from build123d import *


with BuildPart() as f5:
    # F2 (on offset) → F5 section 0
    with BuildSketch(Plane.XY.offset(2), mode=Mode.PRIVATE) as f5_s0:
        Polygon((9.893138, -2.562072), (8.171379, 6.137341), (0.296405, 10.215211), (-7.801768, 6.600819), (-10.025051, -1.984125), (-4.699266, -9.074982), (4.165162, -9.332193), align=None)
    loft([Vertex(0.172753, -0.103171, 12), f5_s0.sketch])

    # F0 (on Top) → F6 section 0
    with BuildSketch(Plane.XY):
        Polygon((7.732626, -1.753436), (6.192105, 4.952361), (-0.011197, 7.928929), (-6.206068, 4.934852), (-7.727643, -1.775269), (-3.430145, -7.148577), (3.450322, -7.13886), align=None)
    # F5_face (on face) → F6 section 1
    with BuildSketch(Plane(origin=(0, 0, 2), x_dir=(1, 0, 0), z_dir=(0, 0, -1))):
        Polygon((9.893138, 2.562072), (4.165162, 9.332193), (-4.699266, 9.074982), (-10.025051, 1.984125), (-7.801768, -6.600819), (0.296405, -10.215211), (8.171379, -6.137341), align=None)
    loft()


solid = f5.part
Geometry: final body of the model. Coordinates: model frame, mm. Round coordinates to 2 decimals unless told otherwise and drop trailing zeros. Loops run counter-clockwise (first coordinate to the right, second up) from the corner with the lowest first, then second, coordinate; pieces in that order, holes last. Notation, with made-up numbers: (-24.75, 1) - (10.25, 1) arc R19 ccw to (10.25, 7) - close; hole circle Ø2 at (-38, 26.5). An arc over 180 degrees is marked (long way). Write each question's results on one line, items separated by ' | '. Start each with the question number.
1) First-contact query: P1, Ø2, axis at x = -3, z = 8.5, coming from the -Y side; P2, Ø2, axis at x = -0.5, y = -1, coming from the +Z side; P3, Ø4, axis at x = 2.5, y = 7, coming from the +Z side. Flat tips, straight axial feed; report the tip coordinate or a pass-through.
2) Cut plane B-B on z = 10.25. Return loops of the section in (x, y), then the cut area to 3 significant figures.
3) Line query: probe 1 along Z at (x, y) = (-5.25, 0.75); probe 2 along X at (y, z) = (-5.25, 1.5); probe 3 along Z at (x, y) = (-3.75, -5). Output: solid intervals per line, ascending. Write a range as [from, to].
4) Cut plane A-A on z = 7. Return loops of the section in (x, y).
5) Mould query, pull axis X, two halves, no side actions, for faces 1 (the face through (0, 0, 0)), 2 (the face through (2.67, 5.02, 5.82)), 3 (the face through (-2.2, 5.2, 5.8)). Classes: released by +X, released by -X, zero draft, split by the parting line, or undercut.
Verdict:
1) P1: stops at y = -3.33 | P2: stops at z = 11.88 | P3: stops at z = 6.17
2) outline: (-1.61, -0.43) - (-0.68, -1.67) - (0.87, -1.72) - (1.87, -0.53) - (1.57, 0.99) - (0.19, 1.7) - (-1.22, 1.07) - close | area: 8.75 mm2
3) probe 1: z = [0, 6.19] | probe 2: x = [-6.93, 6.94] | probe 3: z = [0, 5.45]
4) outline: (-4.93, -1.04) - (-2.26, -4.59) - (2.17, -4.72) - (5.03, -1.33) - (4.17, 3.02) - (0.23, 5.06) - (-3.81, 3.25) - close
5) face 1: zero draft | face 2: released by +X | face 3: released by -X
